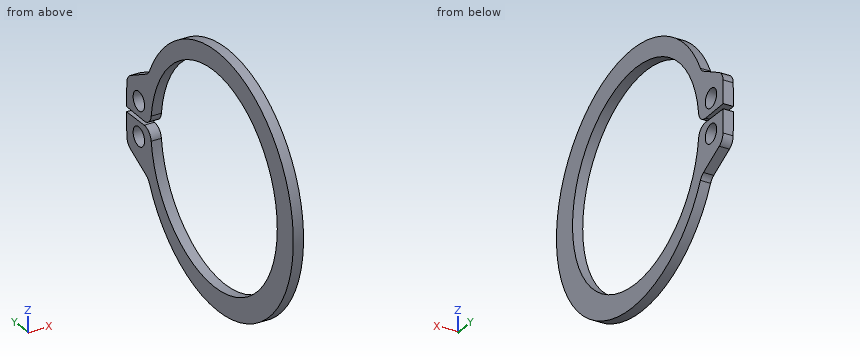
from build123d import *

# Parameters (mm, degrees)
BOSS_EXTRUDE1_DEPTH      = 0.5334
BOSS_EXTRUDE1_DEPTH_BACK = 0.5334
SKETCH3_R                = 0.9906
FILLET1_R                = 1.2065


with BuildPart() as part:
    # Sketch3 → Boss-Extrude1 (new, two sides: drawn at the far end of the back side and taken through both)
    with BuildSketch(Plane(origin=(0, 0, 0), x_dir=(0, 0, -1), z_dir=(1, 0, 0)).offset(-BOSS_EXTRUDE1_DEPTH_BACK)):
        with BuildLine():
            Line((-3.427571395, 15.169791064), (-5.352943643, 11.418661811))
            ThreePointArc((-5.352943643, 11.418661811), (0, -13.8049), (5.352943643, 11.418661811))
            Line((5.352943643, 11.418661811), (3.427571395, 15.169791064))
            Line((3.427571395, 15.169791064), (0.265753029, 15.224980808))
            Line((0.265753029, 15.224980808), (0.192166702, 11.009222987))
            ThreePointArc((0.192166702, 11.009222987), (0, -11.0109), (-0.192166702, 11.009222987))
            Line((-0.192166702, 11.009222987), (-0.265753029, 15.224980808))
            Line((-0.265753029, 15.224980808), (-3.427571395, 15.169791064))
        make_face()
        with Locations((-1.809869048, 13.089507025)):
            Circle(SKETCH3_R, mode=Mode.SUBTRACT)
        with Locations((1.809869048, 13.089507025)):
            Circle(SKETCH3_R, mode=Mode.SUBTRACT)
    extrude(amount=BOSS_EXTRUDE1_DEPTH + BOSS_EXTRUDE1_DEPTH_BACK)

    # Fillet1
    fillet1_edges = [part.edges().sort_by_distance(p)[0] for p in [
        (0, 11.418661811, 5.352943643),
        (0, 15.169791064, 3.427571395),
        (0, 11.009222987, 0.192166702),
        (0, 11.009222987, -0.192166702),
        (0, 15.169791064, -3.427571395),
        (0, 11.418661811, -5.352943643),
    ]]
    fillet(fillet1_edges, radius=FILLET1_R)


solid = part.part
Geometry: final body of the model. Coordinates: model frame, mm. Give positions to 0.01 mm unless a question says otherwise; leave off trailing zeros. Loops run counter-clockwise (first coordinate to the right, second up) from the corner with the lowest first, then second, coordinate; pieces in that order, holes last. Notation, with made-up numbers: (83, 8) -> (122, 8) arc R19 ccw to (122, 44) -> close; hole circle Ø3 at (29, 82.5). An arc over 180 degrees is marked (long way). Put each result on its own line as item: value.
1. Cut plane C-C (x = -0.2). Return the cut outline in (y, z), plus the area to 3 significant figures.
Taken from the geometry:
outline: (10.94, -1.28) arc R11.01 cw (long way) to (10.94, 1.28) arc R1.21 ccw to (12.16, 0.21) -> (15.22, 0.27) -> (15.18, 2.71) arc R1.21 ccw to (14.53, 3.76) -> (11.79, 5.16) arc R1.21 cw to (11.25, 5.71) arc R13.18 ccw (long way) to (11.25, -5.71) arc R1.21 cw to (11.79, -5.16) -> (14.53, -3.76) arc R1.21 ccw to (15.18, -2.71) -> (15.22, -0.27) -> (12.16, -0.21) arc R1.21 ccw to start; hole circle Ø1.98 at (13.09, -1.81); hole circle Ø1.98 at (13.09, 1.81)
area: 181 mm2
2. Cut plane B-B (z = -6.75). Return the cut outline in (x, y).
Taken from the geometry:
outline: (-0.53, -11.95) -> (0.53, -11.95) -> (0.53, -8.7) -> (-0.53, -8.7) -> close; (-0.53, 8.7) -> (0.53, 8.7) -> (0.53, 10.69) -> (-0.53, 10.69) -> close
3. Cut plane A-A (y = -7.75). Return the cut outline in (x, z), plus the area to 3 significant figures.
Taken from the geometry:
outline: (-0.53, -11.09) -> (0.53, -11.09) -> (0.53, -7.82) -> (-0.53, -7.82) -> close; (-0.53, 7.82) -> (0.53, 7.82) -> (0.53, 11.09) -> (-0.53, 11.09) -> close
area: 6.97 mm2
4. Cut plane D-D (z = 1.75). Return the cut outline in (x, y).
Taken from the geometry:
outline: (-0.53, -13.69) -> (0.53, -13.69) -> (0.53, -10.87) -> (-0.53, -10.87) -> close; (-0.53, 10.87) -> (0.53, 10.87) -> (0.53, 12.1) -> (-0.53, 12.1) -> close; (-0.53, 14.08) -> (0.53, 14.08) -> (0.53, 15.2) -> (-0.53, 15.2) -> close
5. Ray query, line 1 along Y through (x, z) = (0.4, -2.5); line 2 along Y through (x, z) = (0, 2.25); line 3 along Y through (x, z) = (0, 6.5). Return the intervals inside material, ascending. Write a range as [from, to].
Taken from the geometry:
line 1: y = [-13.57, -10.72], [10.72, 12.38], [13.8, 15.19]
line 2: y = [-13.61, -10.78], [10.78, 12.2], [13.98, 15.19]
line 3: y = [-12.09, -8.89], [8.89, 10.84]
6. Pin query (flat end, axial travel): P1, Ø2.5, axis at y = 13.09, z = 1.81, coming from the -X side. Return the tip coordinate at first contact, or that it passes through.
Taken from the geometry:
P1: stops at x = -0.53
